Verification items for the finished model (mm, model axes). Face numbers are marked on the shaded views. A direction names the side the tool comes from. Give positions to 0.01 mm unless a question says otherwise; leave off trailing zeros. Order: outer loops, then holes, each group sorted by start corner. A loop starts at its lowest first (then second) coordinate and runs counter-clockwise, first axis right, second up.
(1) Sectioned sample at A-A on z = 0. Record the cut outline in (x, y), plus the area to 3 significant figures.
(2) Sectioned sample at B-B on x = 18. Record the cut outline in (y, z), plus the area to 3 significant figures.
(3) Gauge pin test, flat ends, axial feed: pin 1 (1.5 mm diameter, centred on y = 1.5, z = 6.5, fed in from +X); pin 2 (1.5 mm diameter, centred on x = 1, y = 1.5, fed in from -Z); pin 3 (0.9 mm diameter, centred on x = 1, y = 1, fed in from +Z). Record the tip position at first contact, or that the pin passes through.
(4) Access from +Z, -Z, +X, -X, +Y, -Y to the whole of each face (thin tool, end or side, straight path). Record for the marked faces 1, 2, 3 and 4.
(5) Scan lines: L1, parallel to X at y = 1.7, z = 0; L2, parallel to X at y = 1.4, z = 4.5; L3, parallel to Z at x = 25, y = 0.7. Record each from-to range of solid material in increasing order.
(6) Mould release check, pull along Z, two halves, no side actions. Record for the marked faces 5, 6 and 7: pulls with the +Z half, pulls with the -Z half, needs draft (parallel to the pull), parting line crosses it, or undercut.
(7) Sectioned sample at C-C on y = 1.75. Record the cut outline in (x, z).
```python
from build123d import *

# Parameters (mm, degrees)
CROQUIS1_R              = 7.75
SALIENTE_EXTRUIR1_DEPTH = 3


with BuildPart() as part:
    # Croquis1 → Saliente-Extruir1 (new body)
    with BuildSketch(Plane(origin=(0, 0, 0), x_dir=(1, 0, 0), z_dir=(0, 1, 0))):
        Polygon((0, -5), (0, 5), (3, 5), (3, 10), (33, 10), (33, 5), (36, 5), (36, -5), (33, -5), (33, -10), (3, -10), (3, -5), align=None)
        with Locations(Location((18, 0, 0), (0, 0, 270))):
            Circle(CROQUIS1_R, mode=Mode.SUBTRACT)
    extrude(amount=SALIENTE_EXTRUIR1_DEPTH)


solid = part.part
```
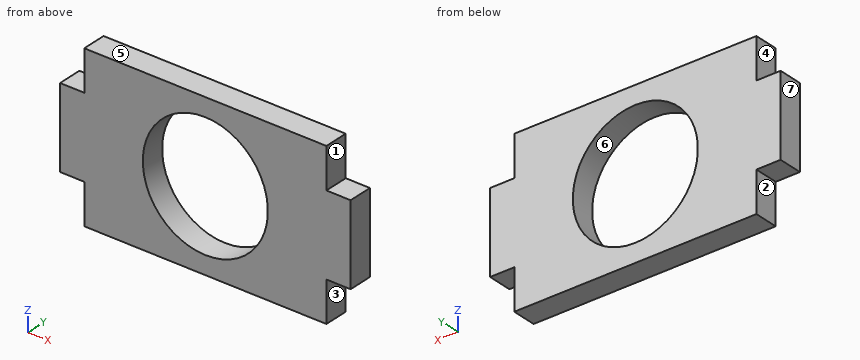
Ans:
1. outline: (0, 0) - (10.25, 0) - (10.25, 3) - (0, 3) - close; (25.75, 0) - (36, 0) - (36, 3) - (25.75, 3) - close
1. area: 61.5 mm2
2. outline: (0, -10) - (3, -10) - (3, -7.75) - (0, -7.75) - close; (0, 7.75) - (3, 7.75) - (3, 10) - (0, 10) - close
2. area: 13.5 mm2
3. pin 1: stops at x = 33
3. pin 2: stops at z = -5
3. pin 3: stops at z = 5
4. face 1: +Z, +X, +Y, -Y
4. face 2: -Z, -X, +Y, -Y
4. face 3: -Z, +X, +Y, -Y
4. face 4: +Z, -X, +Y, -Y
5. L1: x = 0 to 10.25, 25.75 to 36
5. L2: x = 0 to 11.69, 24.31 to 36
5. L3: z = -10 to -3.33, 3.33 to 10
6. face 5: pulls with the +Z half
6. face 6: undercut
6. face 7: needs draft
7. outline: (0, -5) - (3, -5) - (3, -10) - (33, -10) - (33, -5) - (36, -5) - (36, 5) - (33, 5) - (33, 10) - (3, 10) - (3, 5) - (0, 5) - close; hole circle Ø15.5 at (18, 0)
